Input: part model. Units: mm. Frame: model coordinates. Face numbers are marked on the shaded views. Coordinates: 2 decimals unless noted, no trailing zeros. Order: outer loops, then holes, each group sorted by start corner. A loop starts at its lowest first (then second) coordinate and runs counter-clockwise, first axis right, second up. Notation, with made-up numbers: M -31.75,30.5 L 1.25,30.5 A18 cw 1.25,60.5 Z; hole C 3,-28.5 d6. An arc over 180 degrees is marked long. One line per item, written item: value.
```python
from build123d import *

# Parameters (mm, degrees)
SKETCH1_R      = 12.0135
EXTRUDE1_DEPTH = 10
SKETCH3_R      = 8.0045
EXTRUDE2_DEPTH = 8
SKETCH4_R      = 6.5
EXTRUDE3_DEPTH = 19.778934062
FILLET1_R      = 0.25
EXTRUDE4_START = -1.78
SKETCH5_R      = 8.4275
EXTRUDE4_DEPTH = 1.17
EXTRUDE5_REACH = 21.714
SKETCH6_R      = 8.0375
CHAMFER2_SIZE  = 1.5
CHAMFER2_SIZE2 = 0.401923789


with BuildPart() as part:
    # Sketch1 → Extrude1 (new body)
    with BuildSketch(Plane.XY):
        Circle(SKETCH1_R)
    extrude(amount=EXTRUDE1_DEPTH)

    # Sketch3 → Extrude2 (cut)
    with BuildSketch(Plane.XY.offset(10)):
        Circle(SKETCH3_R)
    extrude(amount=-EXTRUDE2_DEPTH, mode=Mode.SUBTRACT)

    # Sketch4 → Extrude3 (cut, through all)
    with BuildSketch(Plane.XY.offset(2)):
        Circle(SKETCH4_R)
    extrude(amount=-EXTRUDE3_DEPTH, mode=Mode.SUBTRACT)

    # Fillet1
    fillet1_edges = [part.edges().sort_by_distance(p)[0] for p in [
        (-8.0045, 0, 2),
    ]]
    fillet(fillet1_edges, radius=FILLET1_R)

    # Sketch5 → Extrude4 (cut)
    with BuildSketch(Plane.XY.offset(10).offset(EXTRUDE4_START)):
        Circle(SKETCH5_R)
    extrude(amount=-EXTRUDE4_DEPTH, mode=Mode.SUBTRACT)

    # Sketch6 → Extrude5 (cut, up to next)
    with BuildSketch(Plane.XY.offset(10), mode=Mode.PRIVATE) as extrude5_sk1:
        Circle(SKETCH6_R)
    extrude5_tool1 = extrude(extrude5_sk1.sketch, amount=-EXTRUDE5_REACH, mode=Mode.PRIVATE) & part.part
    add(extrude5_tool1.solids().sort_by_distance((0, 0, 10))[0], mode=Mode.SUBTRACT)

    # Chamfer2
    chamfer2_edges = [part.edges().sort_by_distance(p)[0] for p in [
        (-12.0135, 0, 10),
    ]]
    chamfer2_side = [part.faces().sort_by_distance(p)[0] for p in [
        (-12.0135, 0, 5),
    ]]
    chamfer(chamfer2_edges, length=CHAMFER2_SIZE, length2=CHAMFER2_SIZE2, reference=chamfer2_side[0])


solid = part.part
```
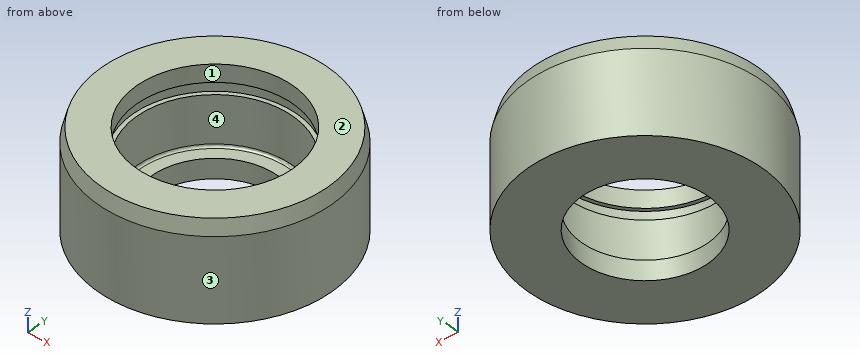
(1) Cut plane A-A on x = 0. Output: boundary loops of the cut face in (y, z).
Data:
outline: M -12.01,0 L -6.5,0 L -6.5,2 L -7.75,2 A0.25 cw -8,2.25 L -8,7.05 L -8.43,7.05 L -8.43,8.22 L -8.04,8.22 L -8.04,10 L -11.61,10 L -12.01,8.5 Z; M 6.5,0 L 12.01,0 L 12.01,8.5 L 11.61,10 L 8.04,10 L 8.04,8.22 L 8.43,8.22 L 8.43,7.05 L 8,7.05 L 8,2.25 A0.25 cw 7.75,2 L 6.5,2 Z
(2) Cut plane C-C on z = 1.25. Output: boundary loops of the cut face in (x, y), plus the area to 3 significant figures.
Data:
outline: C 0,0 d24.03; hole C 0,0 d13
area: 321 mm2
(3) Cut plane D-D on z = 3.25. Output: boundary loops of the cut face in (x, y).
Data:
outline: C 0,0 d24.03; hole C 0,0 d16.01
(4) Ray query, line 1 (Y direction, x = 0, z = 6.5); line 2 (Y direction, x = 0, z = 0.9); line 3 (X direction, y = -6, z = 7.25). Return the intervals inside material, ascending. Write a range as from..to.
Data:
line 1: y = -12.01..-8, 8..12.01
line 2: y = -12.01..-6.5, 6.5..12.01
line 3: x = -10.41..-5.92, 5.92..10.41
(5) Draft query along Y for the marked faces 1, 2, 3 and 4. Return one class per face: released by +Y, released by -Y, zero draft, split by the parting line, or undercut.
Data:
face 1: undercut
face 2: zero draft
face 3: split by the parting line
face 4: undercut
(6) First-contact query: pin 1 (3 mm diameter, centred on y = 4.5, z = 4.5, fed in from +X); pin 2 (3 mm diameter, centred on y = 9.5, z = 8, fed in from -X); pin 3 (1.5 mm diameter, centred on x = -4.5, y = -4, fed in from +Z). Flat tips, straight axial feed; report the tip coordinate or a pass-through.
Data:
pin 1: stops at x = 11.63
pin 2: stops at x = -8.96
pin 3: stops at z = 2
